from build123d import *

# Parameters (mm, degrees)
SKETCH1_W           = 533.4
SKETCH1_H           = 419.1
BOSS_EXTRUDE1_DEPTH = 3.175
SKETCH2_R           = 4.4196
CUT_EXTRUDE1_DEPTH  = 340.235043886
SKETCH3_R           = 8.73125
CUT_EXTRUDE2_DEPTH  = 340.235043886
FILLET1_R           = 12.7
SKETCH5_R           = 1.5367
CUT_EXTRUDE4_DEPTH  = 340.235043886
SKETCH6_R           = 4.7625
CUT_EXTRUDE5_DEPTH  = 340.235043886
SKETCH7_R           = 8.73125
CUT_EXTRUDE6_DEPTH  = 340.235043886


with BuildPart() as part:
    # Sketch1 → Boss-Extrude1 (new, symmetric)
    with BuildSketch(Plane(origin=(0, 0, 0), x_dir=(1, 0, 0), z_dir=(0, 1, 0))):
        Rectangle(SKETCH1_W, SKETCH1_H)
    extrude(amount=BOSS_EXTRUDE1_DEPTH, both=True)

    # Sketch2 → Cut-Extrude1 (cut, through all)
    with BuildSketch(Plane(origin=(0, 3.175, 0), x_dir=(1, 0, 0), z_dir=(0, 1, 0))):
        with Locations(Location((-209.55, -190.5, 0), (0, 0, 270))):
            Circle(SKETCH2_R)
        with Locations(Location((-171.45, -190.5, 0), (0, 0, 270))):
            Circle(SKETCH2_R)
        with Locations(Location((-133.35, -190.5, 0), (0, 0, 270))):
            Circle(SKETCH2_R)
        with Locations(Location((-95.25, -190.5, 0), (0, 0, 270))):
            Circle(SKETCH2_R)
        with Locations(Location((-57.15, -190.5, 0), (0, 0, 270))):
            Circle(SKETCH2_R)
        with Locations(Location((-19.05, -190.5, 0), (0, 0, 270))):
            Circle(SKETCH2_R)
        with Locations(Location((19.05, -190.5, 0), (0, 0, 270))):
            Circle(SKETCH2_R)
        with Locations(Location((-247.65, -190.5, 0), (0, 0, 270))):
            Circle(SKETCH2_R)
        with Locations(Location((57.15, -190.5, 0), (0, 0, 270))):
            Circle(SKETCH2_R)
        with Locations(Location((95.25, -190.5, 0), (0, 0, 270))):
            Circle(SKETCH2_R)
        with Locations(Location((133.35, -190.5, 0), (0, 0, 270))):
            Circle(SKETCH2_R)
        with Locations(Location((171.45, -190.5, 0), (0, 0, 270))):
            Circle(SKETCH2_R)
        with Locations(Location((209.55, -190.5, 0), (0, 0, 270))):
            Circle(SKETCH2_R)
        with Locations(Location((247.65, -190.5, 0), (0, 0, 270))):
            Circle(SKETCH2_R)
        with Locations((285.75, -190.5)):
            Circle(SKETCH2_R)
    extrude(amount=-CUT_EXTRUDE1_DEPTH, mode=Mode.SUBTRACT)

    # Sketch3 → Cut-Extrude2 (cut, through all)
    with BuildSketch(Plane(origin=(0, 3.175, 0), x_dir=(1, 0, 0), z_dir=(0, 1, 0))):
        with Locations(Location((-247.65, -190.5, 0), (0, 0, 270))):
            Circle(SKETCH3_R)
        with Locations(Location((-209.55, -190.5, 0), (0, 0, 270))):
            Circle(SKETCH3_R)
        with Locations(Location((-171.45, -190.5, 0), (0, 0, 270))):
            Circle(SKETCH3_R)
        with Locations(Location((-133.35, -190.5, 0), (0, 0, 270))):
            Circle(SKETCH3_R)
        with Locations(Location((-95.25, -190.5, 0), (0, 0, 270))):
            Circle(SKETCH3_R)
        with Locations(Location((-57.15, -190.5, 0), (0, 0, 270))):
            Circle(SKETCH3_R)
        with Locations(Location((-19.05, -190.5, 0), (0, 0, 270))):
            Circle(SKETCH3_R)
        with Locations(Location((19.05, -190.5, 0), (0, 0, 270))):
            Circle(SKETCH3_R)
        with Locations(Location((57.15, -190.5, 0), (0, 0, 270))):
            Circle(SKETCH3_R)
        with Locations(Location((95.25, -190.5, 0), (0, 0, 270))):
            Circle(SKETCH3_R)
        with Locations(Location((133.35, -190.5, 0), (0, 0, 270))):
            Circle(SKETCH3_R)
        with Locations(Location((171.45, -190.5, 0), (0, 0, 270))):
            Circle(SKETCH3_R)
        with Locations(Location((209.55, -190.5, 0), (0, 0, 270))):
            Circle(SKETCH3_R)
        with Locations(Location((247.65, -190.5, 0), (0, 0, 270))):
            Circle(SKETCH3_R)
        with Locations((285.75, -190.5)):
            Circle(SKETCH3_R)
    extrude(amount=-CUT_EXTRUDE2_DEPTH, mode=Mode.SUBTRACT)

    # Fillet1
    fillet1_edges = [part.edges().sort_by_distance(p)[0] for p in [
        (266.7, 0, 209.55),
        (-266.7, 0, 209.55),
        (-266.7, 0, -209.55),
        (266.7, 0, -209.55),
    ]]
    fillet(fillet1_edges, radius=FILLET1_R)

    # Sketch5 → Cut-Extrude4 (cut, through all)
    with BuildSketch(Plane(origin=(0, 3.175, 0), x_dir=(1, 0, 0), z_dir=(0, 1, 0))):
        with Locations(Location((-215.9, 158.75, 0), (0, 0, 270))):
            Circle(SKETCH5_R)
        with Locations(Location((215.9, 158.75, 0), (0, 0, 270))):
            Circle(SKETCH5_R)
        with Locations(Location((215.9, -158.75, 0), (0, 0, 270))):
            Circle(SKETCH5_R)
        with Locations(Location((-215.9, -158.75, 0), (0, 0, 270))):
            Circle(SKETCH5_R)
    extrude(amount=-CUT_EXTRUDE4_DEPTH, mode=Mode.SUBTRACT)

    # Sketch6 → Cut-Extrude5 (cut, through all)
    with BuildSketch(Plane(origin=(0, 3.175, 0), x_dir=(1, 0, 0), z_dir=(0, 1, 0))):
        with Locations(Location((-10.31875, 38.815634586, 0), (0, 0, 270))):
            Circle(SKETCH6_R)
        with Locations(Location((10.31875, 38.815634586, 0), (0, 0, 270))):
            Circle(SKETCH6_R)
    extrude(amount=-CUT_EXTRUDE5_DEPTH, mode=Mode.SUBTRACT)

    # Sketch7 → Cut-Extrude6 (cut, through all)
    with BuildSketch(Plane(origin=(0, 3.175, 0), x_dir=(1, 0, 0), z_dir=(0, 1, 0))):
        with Locations(Location((-103.272945392, 25.345250482, 0), (0, 0, 270))):
            Circle(SKETCH7_R)
        with Locations(Location((-130.213713756, -1.595517881, 0), (0, 0, 270))):
            Circle(SKETCH7_R)
        with Locations(Location((-53.881536726, -77.92769491, 0), (0, 0, 270))):
            Circle(SKETCH7_R)
        with Locations(Location((-26.940768363, -50.986926547, 0), (0, 0, 270))):
            Circle(SKETCH7_R)
        with Locations(Location((26.940768363, -50.986926547, 0), (0, 0, 270))):
            Circle(SKETCH7_R)
        with Locations(Location((53.881536726, -77.92769491, 0), (0, 0, 270))):
            Circle(SKETCH7_R)
        with Locations(Location((130.213713756, -1.595517881, 0), (0, 0, 270))):
            Circle(SKETCH7_R)
        with Locations(Location((103.272945392, 25.345250482, 0), (0, 0, 270))):
            Circle(SKETCH7_R)
    extrude(amount=-CUT_EXTRUDE6_DEPTH, mode=Mode.SUBTRACT)


solid = part.part
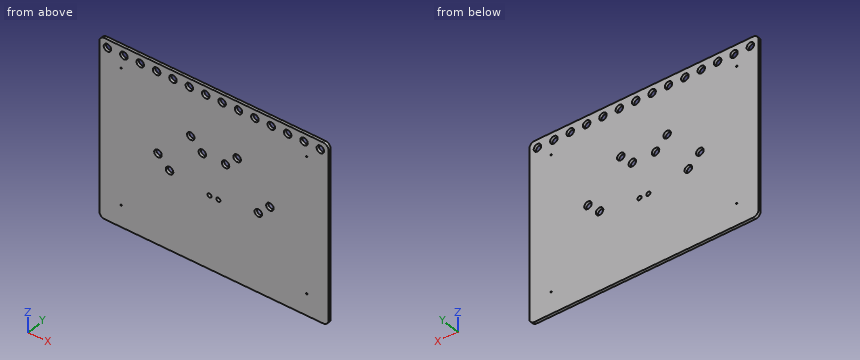
The listing builds one solid part. Answer for the finished solid, in the listing's coordinates (mm). Coordinates: 2 decimals unless noted, no trailing zeros. Order: outer loops, then holes, each group sorted by start corner. A loop starts at its lowest first (then second) coordinate and runs counter-clockwise, first axis right, second up.
Q1. Consider line 1 (X direction, y = -1.75, z = 83); line 2 (X direction, y = -0.5, z = -42); line 3 (Z direction, x = 216.5, y = 1.75). Determine where each line is inside the solid, lowest interval first.
Q2. Given P1, Ø3.5, axis at x = 215.9, z = 158.75, coming from the +Y side (3 decimals), flat-ended and moving along its own axis, determine where the tip first touches the part or whether it passes through.
Q3. A cutting plane is placed at B-B, the plane z = -25. Write down the section's boundary in (x, y) (3 decimals).
Q4. A cutting plane is placed at A-A, the plane x = 247.65. Write down the section's boundary in (y, z) (3 decimals).
Q5. A cutting plane is placed at C-C, the plane y = 0.5. State how many separate pieces and enclosed holes the cut face has, and give its area (3 significant figures).
Answers follow:
1. line 1: x = -266.7 to -60.99, -46.77 to 46.77, 60.99 to 266.7
1. line 2: x = -266.7 to -13.86, -6.78 to 6.78, 13.86 to 266.7
1. line 3: z = -209.55 to -160.16, -157.34 to 157.34, 160.16 to 185.21, 195.79 to 209.55
2. P1: stops at y = 3.175
3. outline: (-266.7, -3.175) - (-111.997, -3.175) - (-111.997, 3.175) - (-266.7, 3.175) - close; (-94.549, -3.175) - (94.549, -3.175) - (94.549, 3.175) - (-94.549, 3.175) - close; (111.997, -3.175) - (266.7, -3.175) - (266.7, 3.175) - (111.997, 3.175) - close
4. outline: (-3.175, -209.55) - (3.175, -209.55) - (3.175, 181.769) - (-3.175, 181.769) - close; (-3.175, 199.231) - (3.175, 199.231) - (3.175, 209.55) - (-3.175, 209.55) - close
5. separate pieces: 1
5. enclosed holes: 28
5. area: 218,000 mm2
